from build123d import *

# Parameters (mm, degrees)
EXTRUDE1_DEPTH      = 1.5
EXTRUDE1_DEPTH_BACK = 3.5
SKETCH2_R           = 2.656835516
EXTRUDE2_DEPTH      = 13.5


with BuildPart() as part:
    # Sketch1 → Extrude1 (new, two sides: drawn at the far end of the back side and taken through both)
    with BuildSketch(Plane.XY.offset(-EXTRUDE1_DEPTH_BACK)):
        Polygon((-2.458590949, 104.784469075), (-4.658295474, 108.594469075), (-9.057704526, 108.594469075), (-11.257409051, 104.784469075), (-9.057704526, 100.974469075), (-4.658295474, 100.974469075), align=None)
    extrude(amount=EXTRUDE1_DEPTH + EXTRUDE1_DEPTH_BACK)

    # Sketch2 → Extrude2 (add)
    with BuildSketch(Plane.XY.offset(1.5)):
        with Locations(Location((-6.858, 104.784469075, 0), (0, 0, 180))):
            Circle(SKETCH2_R)
    extrude(amount=EXTRUDE2_DEPTH)


solid = part.part
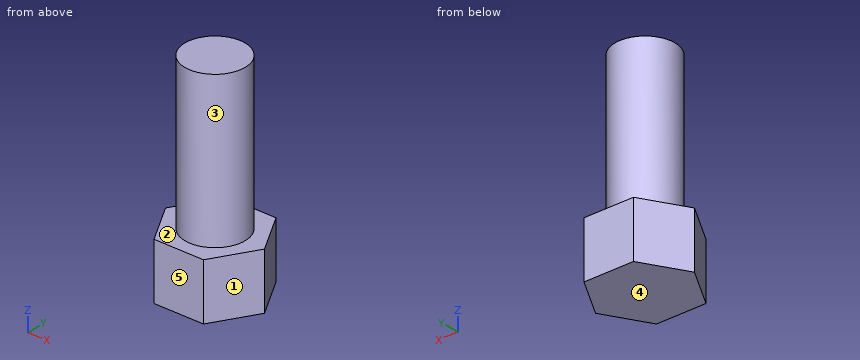
Can you work these out from the model? Positions are in its coordinate system, mm. Face numbers are marked on the shaded views. A direction names the side the tool comes from. Give positions to 0.01 mm unless a question says otherwise; leave off trailing zeros. Order: outer loops, then holes, each group sorted by start corner. A loop starts at its lowest first (then second) coordinate and runs counter-clockwise, first axis right, second up. Notation, with made-up numbers: (-8.5, -16.5) - (32.5, -16.5) arc R16 ccw to (32.5, -12.5) - close; hole circle Ø9 at (66.25, -7.5). An arc over 180 degrees is marked (long way). Write each question's results on one line, items separated by ' | '.
1) If we mould it in two halves opening along Y, with no side actions, what happens to the marked faces 3, 4 and 5? For each: pulls with the +Y half, pulls with the -Y half, needs draft (parallel to the pull), parting line crosses it, or undercut.
Final values:
face 3: parting line crosses it | face 4: needs draft | face 5: pulls with the -Y half
2) Please list where these lines run through material, in increasing order: line 1 along X through (y, z) = (104.75, 8.25); line 2 along Z through (x, y) = (-6.25, 101.75); line 3 along X through (y, z) = (105, -1.5). Write a range as [from, to].
Final values:
line 1: x = [-9.51, -4.2] | line 2: z = [-3.5, 1.5] | line 3: x = [-11.13, -2.58]
3) Suppose I cut it at C-C, the plane z = 1. Write out the boundary of the cut face in (x, y), then the cut area to 3 significant figures.
Final values:
outline: (-11.26, 104.78) - (-9.06, 100.97) - (-4.66, 100.97) - (-2.46, 104.78) - (-4.66, 108.59) - (-9.06, 108.59) - close | area: 50.3 mm^2
4) Suppose I cut it at D-D, the plane z = 7.25. Write out the boundary of the cut face in (x, y).
Final values:
outline: circle Ø5.31 at (-6.86, 104.78)
5) Suppose I cut it at B-B, the plane y = 102.5. Write out the boundary of the cut face in (x, z), then the cut area to 3 significant figures.
Final values:
outline: (-9.94, -3.5) - (-3.78, -3.5) - (-3.78, 1.5) - (-5.5, 1.5) - (-5.5, 15) - (-8.21, 15) - (-8.21, 1.5) - (-9.94, 1.5) - close | area: 67.4 mm^2
6) On a 3-axis mill with a long thin cutter (end or side, diameter ignored), from which of +Z, -Z, +X, -X, +Y, -Y can I reach the whole of each face in a straight line? I mean the marked faces 1 and 2. Say none if no direction works.
Final values:
face 1: +Z, -Z, +X, -Y | face 2: +Z
7) Suppose I cut it at A-A, the plane x = -8. Write out the boundary of the cut face in (y, z).
Final values:
outline: (100.97, -3.5) - (108.59, -3.5) - (108.59, 1.5) - (107.18, 1.5) - (107.18, 15) - (102.39, 15) - (102.39, 1.5) - (100.97, 1.5) - close
8) I'm going to push flat-ended pins straight in: pin 1 Ø2 at (x, z) = (-7, 12) entering from +Y; pin 2 Ø3 at (x, z) = (-4.5, 6.5) entering from -Y; pin 3 Ø1.5 at (y, z) = (107.5, -1) entering from -X. Where does each tip first touch, or does it pass through?
Final values:
pin 1: stops at y = 107.44 | pin 2: stops at y = 102.27 | pin 3: stops at x = -10.12
